```python
from build123d import *

# Parameters (mm, degrees)
SKETCH1_W           = 80
SKETCH1_H           = 40
BOSS_EXTRUDE1_DEPTH = 2.5
SKETCH3_R           = 6
BOSS_EXTRUDE2_DEPTH = 2.5


with BuildPart() as part:
    # Sketch1 → Boss-Extrude1 (new body)
    with BuildSketch(Plane(origin=(0, 0, 0), x_dir=(1, 0, 0), z_dir=(0, 1, 0))):
        with Locations((40, 20)):
            Rectangle(SKETCH1_W, SKETCH1_H)
    extrude(amount=BOSS_EXTRUDE1_DEPTH)

    # Sketch3 → Boss-Extrude2 (add)
    with BuildSketch(Plane(origin=(0, 0, -40), x_dir=(-1, 0, 0), z_dir=(0, 0, -1))):
        with BuildLine():
            ThreePointArc((0, 2.5), (-0.57985041, 6.339255677), (-2.267674485, 9.836019972))
            Line((-2.267674485, 9.836019972), (-29.267674485, 49.336019972))
            ThreePointArc((-29.267674485, 49.336019972), (-40, 55), (-50.732325515, 49.336019972))
            Line((-50.732325515, 49.336019972), (-77.732325515, 9.836019972))
            ThreePointArc((-77.732325515, 9.836019972), (-79.42014959, 6.339255677), (-80, 2.5))
            Line((-80, 2.5), (0, 2.5))
        make_face()
        with Locations((-40, 42)):
            Circle(SKETCH3_R, mode=Mode.SUBTRACT)
    extrude(amount=-BOSS_EXTRUDE2_DEPTH)


solid = part.part
```
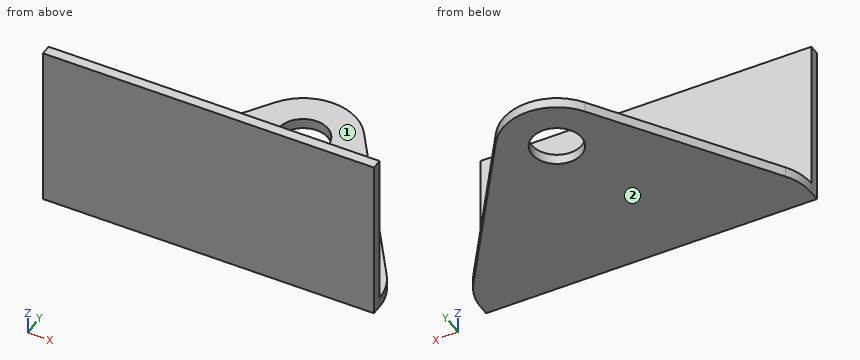
Geometry: final body of the model. Coordinates: model frame, mm. Face numbers are marked on the shaded views. A direction names the side the tool comes from. Coordinates: 2 decimals unless noted, no trailing zeros. Order: outer loops, then holes, each group sorted by start corner. A loop starts at its lowest first (then second) coordinate and runs counter-clockwise, first axis right, second up. Notation, with made-up numbers: (27.5, 59.25) -> (36.5, 59.25) arc R12 cw to (36.5, 69.25) -> close; hole circle Ø8 at (46.25, 36.25). An arc over 180 degrees is marked (long way). Write each question's results on one line, items separated by ' | '. Start each with the question number.
1) First-contact query: pin 1 (4 mm diameter, centred on x = 36, y = 12, fed in from +Z); pin 2 (11 mm diameter, centred on x = 29, z = -14, fed in from +Y). Flat tips, straight axial feed; report the tip coordinate or a pass-through.
2) Material intervals for line 1 along Y through (x, z) = (40, -38); line 2 along Y through (x, z) = (30, -20.5); line 3 along Z through (x, y) = (25.5, 12), sorted ascending.
3) Cut plane B-B, the plane y = 42. Output: boundary loops of the cut face in (x, z).
4) Set-up query: the marked faces 1 and 2. Return all of +Z, -Z, +X, -X, +Y, -Y with unobstructed straight access to the full face (end or side cutting, diameter ignored); none if empty.
5) Cut plane C-C, the plane z = -12.5. Output: boundary loops of the cut face in (x, y), and give its area (3 significant figures).
6) Cut plane A-A, the plane x = 40. Output: boundary loops of the cut face in (y, z), and give its area (3 significant figures).
7) Cut plane D-D, the plane x = 7. Output: boundary loops of the cut face in (y, z), and give its area (3 significant figures).
Checks:
1) pin 1: z = -37.5 | pin 2: y = 2.5
2) line 1: 0 to 36, 48 to 55 | line 2: 0 to 2.5 | line 3: -40 to -37.5
3) outline: (24.25, -40) -> (34, -40) -> (34, -37.5) -> (24.25, -37.5) -> close; (46, -40) -> (55.75, -40) -> (55.75, -37.5) -> (46, -37.5) -> close
4) face 1: +Z, +X, -X, +Y | face 2: -Z, +X, -X, +Y, -Y
5) outline: (0, 0) -> (80, 0) -> (80, 2.5) -> (0, 2.5) -> close | area: 200 mm^2
6) outline: (0, -40) -> (36, -40) -> (36, -37.5) -> (2.5, -37.5) -> (2.5, 0) -> (0, 0) -> close; (48, -40) -> (55, -40) -> (55, -37.5) -> (48, -37.5) -> close | area: 201 mm^2
7) outline: (0, -40) -> (16.76, -40) -> (16.76, -37.5) -> (2.5, -37.5) -> (2.5, 0) -> (0, 0) -> close | area: 136 mm^2
